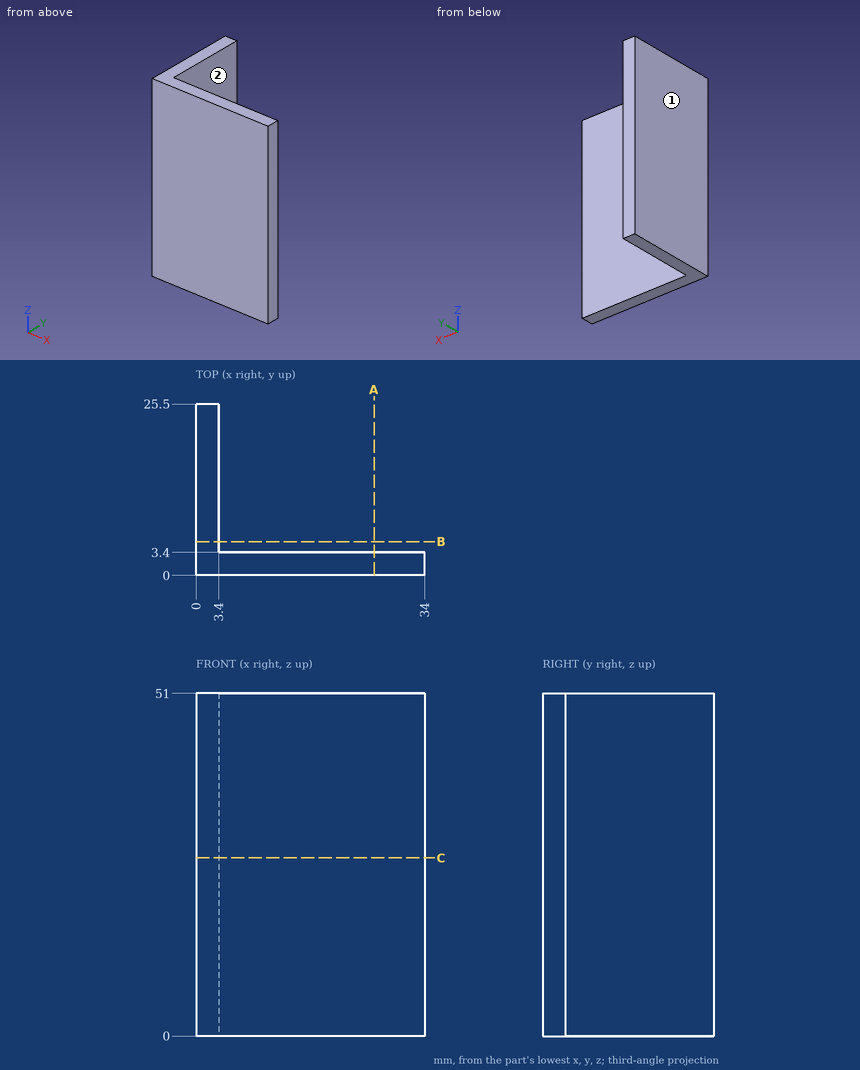
The drawing under review shows one solid part. Ordinate dimensions are in mm from its lowest x, y, z. A direction names the side the tool comes from. Coordinates: 2 decimals unless noted, no trailing zeros. Loops run counter-clockwise (first coordinate to the right, second up) from the corner with the lowest first, then second, coordinate; pieces in that order, holes last. Notation, with made-up numbers: (43.5, 58.25) -> (64.5, 58.25) arc R29 cw to (64.5, 87.25) -> close; hole circle Ø9 at (63.5, -10). An arc over 180 degrees is marked (long way). Answer as a JSON object with one key per item and string values.
Q1. Take a section at A-A on x = 26.5. Give the boundary of the cut face in (y, z).
Answer block:
{"outline": "(0, 0) -> (3.4, 0) -> (3.4, 51) -> (0, 51) -> close"}
Q2. To check wall thickness, follow L1, parallel to X at y = 12.25, z = 34.5. State the ranges of the line that lie inside material, in increasing order.
Answer block:
{"L1": "x = 0 to 3.4"}
Q3. Take a section at C-C on z = 26.5. Give the boundary of the cut face in (x, y), plus the area to 3 significant figures.
Answer block:
{"outline": "(0, 0) -> (34, 0) -> (34, 3.4) -> (3.4, 3.4) -> (3.4, 25.5) -> (0, 25.5) -> close", "area": "191 mm^2"}
Q4. Clearance check with flat-ended pins moving along their axes: pin 1 Ø9 at (x, z) = (23, 36) entering from +Y; pin 2 Ø8 at (y, z) = (22.5, 44) entering from +X; pin 3 Ø10 at (x, y) = (15, 11.5) entering from +Z. State where each tip first meets the part, or that it passes through.
Answer block:
{"pin 1": "stops at y = 3.4", "pin 2": "stops at x = 3.4", "pin 3": "passes through"}
Q5. Tool access review of the marked faces 1 and 2: name each direction out of +Z, -Z, +X, -X, +Y, -Y from which nothing blocks a thin tool from reaching the whole face with its end or side.
Answer block:
{"face 1": "+Z, -Z, -X, +Y, -Y", "face 2": "+Z, -Z, +X, +Y"}
